The model under review builds one solid part; all positions refer to its coordinate system, in mm. Give positions to 0.01 mm unless a question says otherwise; leave off trailing zeros. Order: outer loops, then holes, each group sorted by start corner. A loop starts at its lowest first (then second) coordinate and runs counter-clockwise, first axis right, second up. Notation, with made-up numbers: (42, -7) - (50, -7) arc R26 cw to (50, 8) - close; hole circle Ø10 at (17, 18.25). An arc over 180 degrees is marked (long way). Use CSV: the item, a comma, the result in double quotes.
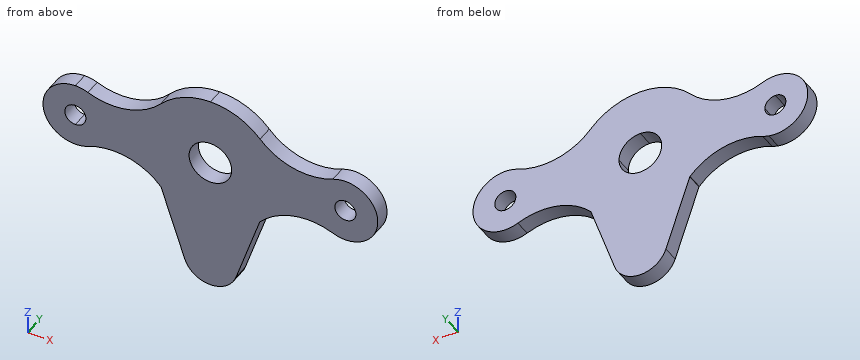
```python
from build123d import *

# Parameters (mm, degrees)
F0_R     = 1.95
F1_DEPTH = 3


with BuildPart() as f1:
    # F0 (on Front) → F1 (new body)
    with BuildSketch(Plane.XZ):
        with BuildLine():
            ThreePointArc((9.196429, 8.46615), (5.021111, 11.447202), (0, 12.5))
            ThreePointArc((0, 12.5), (-5.021111, 11.447202), (-9.196429, 8.46615))
            ThreePointArc((-9.196429, 8.46615), (-15.471851, 4.868407), (-22.675, 5.531218))
            ThreePointArc((-22.675, 5.531218), (-23.814106, 5.881637), (-25, 6))
            ThreePointArc((-25, 6), (-30.968842, -0.610671), (-23.785, -5.875694))
            ThreePointArc((-23.785, -5.875694), (-23.22164, -5.730396), (-22.675, -5.531218))
            ThreePointArc((-22.675, -5.531218), (-15.471851, -4.868407), (-9.196429, -8.46615))
            ThreePointArc((-9.196429, -8.46615), (-9.170756, -8.493952), (-9.145, -8.521677))
            ThreePointArc((-9.145, -8.521677), (-9.145117, -8.521895), (-9.145235, -8.522114))
            Line((-9.145235, -8.522114), (-4.73808, -21.597059))
            ThreePointArc((-4.73808, -21.597059), (0, -25), (4.73808, -21.597059))
            Line((4.73808, -21.597059), (9.145235, -8.522114))
            ThreePointArc((9.145235, -8.522114), (15.434808, -4.876534), (22.675, -5.531218))
            ThreePointArc((22.675, -5.531218), (31, 0), (22.675, 5.531218))
            ThreePointArc((22.675, 5.531218), (15.471851, 4.868407), (9.196429, 8.46615))
        make_face()
        with BuildLine():
            ThreePointArc((-25, -1.95), (-26.95, 0), (-25, 1.95))
            ThreePointArc((-25, 1.95), (-23.621142, 1.378858), (-23.05, 0))
            ThreePointArc((-23.05, 0), (-23.621142, -1.378858), (-25, -1.95))
        make_face(mode=Mode.SUBTRACT)
        with BuildLine():
            ThreePointArc((0, 3.95), (2.793072, 2.793072), (3.95, 0))
            ThreePointArc((3.95, 0), (-2.793072, -2.793072), (0, 3.95))
        make_face(mode=Mode.SUBTRACT)
        with Locations((25, 0)):
            Circle(F0_R, mode=Mode.SUBTRACT)
    extrude(amount=F1_DEPTH)


solid = f1.part
```
Item 1: Take a section at A-A, the plane x = 25. Give the boundary of the cut face in (y, z), and give its area (3 significant figures).
Results list:
outline,"(-3, -6) - (0, -6) - (0, -1.95) - (-3, -1.95) - close; (-3, 1.95) - (0, 1.95) - (0, 6) - (-3, 6) - close"
area,"24.3 mm2"
Item 2: Clearance check with flat-ended pins moving along their axes: pin 1 (2.5 mm diameter, centred on x = 25, z = 0, fed in from -Y); pin 2 (1 mm diameter, centred on y = -0.5, z = -2, fed in from -X); pin 3 (1 mm diameter, centred on y = -1, z = -19.5, fed in from -X). State where each tip first meets the part, or that it passes through.
Results list:
pin 1,"passes through"
pin 2,"stops at x = -30.81"
pin 3,"stops at x = -5.61"
Item 3: Take a section at B-B, the plane y = -0.5. State how many separate pieces and enclosed holes the cut face has, and give its area (3 significant figures).
Results list:
separate pieces,"1"
enclosed holes,"3"
area,"959 mm2"
Item 4: Take a section at C-C, the plane z = 10. Give the boundary of the cut face in (x, y), and give its area (3 significant figures).
Results list:
outline,"(-7.5, -3) - (7.5, -3) - (7.5, 0) - (-7.5, 0) - close"
area,"45.0 mm2"
Item 5: Take a section at D-D, the plane x = -16.5. Give the boundary of the cut face in (y, z).
Results list:
outline,"(-3, -4.69) - (0, -4.69) - (0, 4.69) - (-3, 4.69) - close"
Item 6: Wall thickness on L1, parallel to Z at x = 25, y = -1.95; L2, parallel to X at y = -2.4, z = 3; L3, parallel to Z at x = 18, y = -1: over which ranges is each line inside the solid? List them lowest first.
Results list:
L1,"z = -6 to -1.95, 1.95 to 6"
L2,"x = -30.2 to -2.57, 2.57 to 30.2"
L3,"z = -4.59 to 4.59"
